Part print with two shaded views. Sizes in mm from the minimum x, y, z corner. Give positions to 0.01 mm unless a question says otherwise; leave off trailing zeros. Order: outer loops, then holes, each group sorted by start corner. A loop starts at its lowest first (then second) coordinate and runs counter-clockwise, first axis right, second up. Notation, with made-up numbers: (69.25, -4) -> (75.25, -4) arc R29 cw to (75.25, 31) -> close; hole circle Ø5 at (69, -16). An arc over 180 degrees is marked (long way). Answer as CSV lines item,"result".
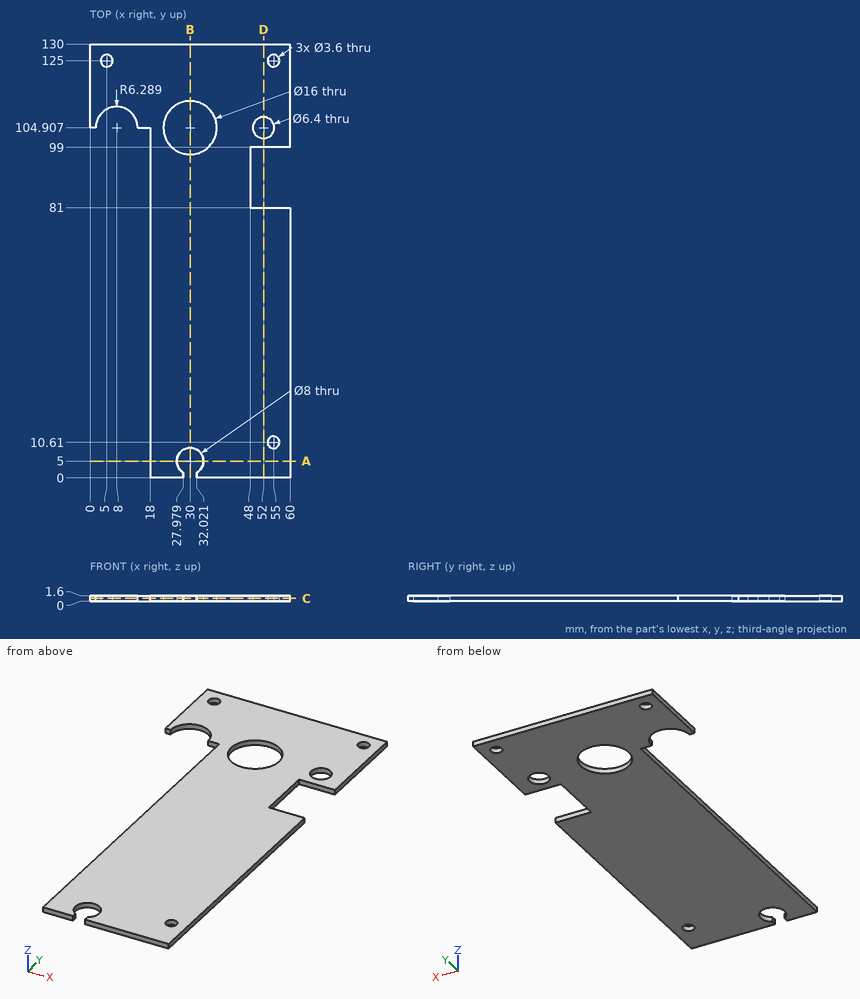
1) Band-saw the part on B-B, the plane x = 30. Write the cut outline in (y, z), then the cut area to 3 significant figures.
Data:
outline,"(9, 0) -> (96.91, 0) -> (96.91, 1.6) -> (9, 1.6) -> close; (112.91, 0) -> (130, 0) -> (130, 1.6) -> (112.91, 1.6) -> close"
area,"168 mm2"
2) Band-saw the part on A-A, the plane y = 5. Write the cut outline in (x, z).
Data:
outline,"(18, 0) -> (26, 0) -> (26, 1.6) -> (18, 1.6) -> close; (34, 0) -> (60, 0) -> (60, 1.6) -> (34, 1.6) -> close"
3) Pin check, flat tips, straight feed: P1, Ø3, axis at x = 55, y = 10.61, coming from the +Z side; P2, Ø0.5, axis at y = 1, z = 0.5, coming from the -X side; P3, Ø0.5, axis at x = 1, z = 0.5, coming from the -Y side. Stop position of each tip, or through.
Data:
P1,"passes through"
P2,"stops at x = 18"
P3,"stops at y = 104.91"
4) Band-saw the part on D-D, the plane x = 52. Write the cut outline in (y, z).
Data:
outline,"(0, 0) -> (81, 0) -> (81, 1.6) -> (0, 1.6) -> close; (99, 0) -> (101.71, 0) -> (101.71, 1.6) -> (99, 1.6) -> close; (108.11, 0) -> (130, 0) -> (130, 1.6) -> (108.11, 1.6) -> close"
5) Band-saw the part on C-C, the plane z = 0.85. Write the cut outline in (x, y).
Data:
outline,"(0, 104.91) -> (1.71, 104.91) arc R6.29 cw to (14.29, 104.91) -> (18, 104.91) -> (18, 0) -> (27.98, 0) -> (27.98, 1.55) arc R4 cw (long way) to (32.02, 1.55) -> (32.02, 0) -> (60, 0) -> (60, 81) -> (48, 81) -> (48, 99) -> (60, 99) -> (60, 130) -> (0, 130) -> close; hole circle Ø3.6 at (5, 125); hole circle Ø16 at (30, 104.91); hole circle Ø6.4 at (52, 104.91); hole circle Ø3.6 at (55, 10.61); hole circle Ø3.6 at (55, 125)"
6) Wall check: line 1 along Y through (x, z) = (30, 1.3); line 2 along Y through (x, z) = (33, 1.55) (1 decimal); line 3 along Y through (x, z) = (50, 0.9) (1 decimal). Give the ranges that are in metal, low to high. Write a range as [from, to].
Data:
line 1,"y = [9, 96.91], [112.91, 130]"
line 2,"y = [0, 2.4], [7.6, 97.5], [112.3, 130]"
line 3,"y = [0, 81], [99, 102.4], [107.4, 130]"
